For this review, take the finished solid that the model builds, in its own axes (mm). A direction names the side the tool comes from. Give positions to 0.01 mm unless a question says otherwise; leave off trailing zeros. Order: outer loops, then holes, each group sorted by start corner. A loop starts at its lowest first (then second) coordinate and runs counter-clockwise, first axis right, second up. Notation, with made-up numbers: (-35.5, -12) -> (-13.5, -12) arc R21 ccw to (-13.5, 10) -> close; hole circle Ø3 at (88, 59.25). An arc over 180 degrees is marked (long way). Return JSON: item names as keys, results as strings. Group by question number.
1) Add section D-D (x = -3.5). Give the boundary of the cut face in (y, z).
2) For faces 5 (the face through (-9.6, 0.07, 1.97)), 6 (the face through (5, -8, 2)), list the 3-axis set-ups (+Z, -Z, +X, -X, +Y, -Y) from which the entire face can be reached by the end or side of a thin tool; tool diameter is ignored.
3) Add section B-B (z = 3.35). Give the boundary of the cut face in (x, y), then the cut area to 3 significant figures.
4) The part is to be moulded in two halves that separate along Y. For faces 1 (the face through (0, 105, 2)), 2 (the face through (-0.35, 6.44, 1.97)), 3 (the face through (6.4, 0.07, 1.97)), 4 (the face through (-13, 44, 2)), say which applies: released by +Y, released by -Y, zero draft, split by the parting line, or undercut.
5) Add section C-C (x = -8). Give the boundary of the cut face in (y, z), then the cut area to 3 significant figures.
6) Add section A-A (y = 8). Give the boundary of the cut face in (x, z), then the cut area to 3 significant figures.
7) Insertion check: P1, Ø2.5, axis at x = -8, y = 0, coming from the +Z side. The pin has a flat end and moves straight along its axis. Give the tip position at first contact, or say it passes through.
8) To check wall thickness, follow line 1 along Y through (x, z) = (0, 1.15); line 2 along Y through (x, z) = (-8, 1.2); line 3 along Y through (x, z) = (-3, 1.9). State the ranges of each line that lie inside material, in increasing order.
from build123d import *

# Parameters (mm, degrees)
SKETCH_1_R      = 1.6
EXTRUDE_1_DEPTH = 4


with BuildPart() as part:
    # 草图1 → 凸台-拉伸1 (new body)
    with BuildSketch(Plane.XY):
        with BuildLine():
            Line((-8, -15), (-13, -15))
            Line((-13, -15), (-13, -12))
            Line((-13, -12), (-13, 105))
            Line((-13, 105), (-11, 105))
            Line((-11, 105), (11, 105))
            Line((11, 105), (13, 105))
            Line((13, 105), (13, -12))
            Line((13, -12), (13, -15))
            Line((13, -15), (8, -15))
            Line((8, -15), (5, -15))
            Line((5, -15), (5, 0))
            ThreePointArc((5, 0), (0, 5), (-5, 0))
            Line((-5, 0), (-5, -15))
            Line((-5, -15), (-8, -15))
        make_face()
        with Locations((8, 0)):
            Circle(SKETCH_1_R, mode=Mode.SUBTRACT)
        with Locations((-8, 0)):
            Circle(SKETCH_1_R, mode=Mode.SUBTRACT)
        with Locations((0, 8)):
            Circle(SKETCH_1_R, mode=Mode.SUBTRACT)
    extrude(amount=EXTRUDE_1_DEPTH)


solid = part.part
Evaluation:
{
 "1": {"outline": "(3.57, 0) -> (105, 0) -> (105, 4) -> (3.57, 4) -> close"},
 "2": {"face 5": "+Z, -Z", "face 6": "+Z, -Z, -Y"},
 "3": {"outline": "(-13, -15) -> (-5, -15) -> (-5, 0) arc R5 cw to (5, 0) -> (5, -15) -> (13, -15) -> (13, 105) -> (-13, 105) -> close; hole circle Ø3.2 at (-8, 0); hole circle Ø3.2 at (0, 8); hole circle Ø3.2 at (8, 0)", "area": "2,910 mm^2"},
 "4": {"face 1": "released by +Y", "face 2": "undercut", "face 3": "undercut", "face 4": "zero draft"},
 "5": {"outline": "(-15, 0) -> (-1.6, 0) -> (-1.6, 4) -> (-15, 4) -> close; (1.6, 0) -> (105, 0) -> (105, 4) -> (1.6, 4) -> close", "area": "467 mm^2"},
 "6": {"outline": "(-13, 0) -> (-1.6, 0) -> (-1.6, 4) -> (-13, 4) -> close; (1.6, 0) -> (13, 0) -> (13, 4) -> (1.6, 4) -> close", "area": "91.2 mm^2"},
 "7": {"P1": "through"},
 "8": {"line 1": "5 to 6.4, 9.6 to 105", "line 2": "-15 to -1.6, 1.6 to 105", "line 3": "4 to 105"}
}
